```python
from build123d import *

# Parameters (mm, degrees)
MODEL_R                 = 1.25
BOSS_EXTRUDE1_DEPTH     = 2
BOSS_EXTRUDE2_DEPTH     = 11.50072
SKETCH2_R               = 1.25
CUT_EXTRUDE1_DEPTH      = 2
CUT_EXTRUDE1_DEPTH_BACK = 4


with BuildPart() as part:
    # Model → Boss-Extrude1 (new body)
    with BuildSketch(Plane.XY):
        Polygon((1.25, 4), (0, 4), (0, 8), (1.25, 8), (1.25, 12), (10.25072, 12), (10.25072, 8), (11.50072, 8), (11.50072, 4), (10.25072, 4), (10.25072, 0), (1.25, 0), align=None)
        with Locations((7.75072, 6)):
            Circle(MODEL_R, mode=Mode.SUBTRACT)
        with Locations((3.75, 6)):
            Circle(MODEL_R, mode=Mode.SUBTRACT)
    extrude(amount=BOSS_EXTRUDE1_DEPTH)

    # Sketch1 → Boss-Extrude2 (add)
    with BuildSketch(Plane.ZY):
        with BuildLine():
            Line((2, 4), (2, 5))
            ThreePointArc((2, 5), (2.292893219, 4.292893219), (3, 4))
            Line((3, 4), (2, 4))
        make_face()
        with BuildLine():
            Line((0, 4), (-1, 4))
            ThreePointArc((-1, 4), (-0.292893219, 4.292893219), (0, 5))
            Line((0, 5), (0, 4))
        make_face()
    extrude(amount=-BOSS_EXTRUDE2_DEPTH)

    # Sketch2 → Cut-Extrude1 (cut, two sides)
    with BuildSketch(Plane.XY.offset(2)) as cut_extrude1_sk:
        with Locations((3.75, 6)):
            Circle(SKETCH2_R)
        with Locations((7.75072, 6)):
            Circle(SKETCH2_R)
    extrude(amount=CUT_EXTRUDE1_DEPTH, mode=Mode.SUBTRACT)
    extrude(cut_extrude1_sk.sketch, amount=-CUT_EXTRUDE1_DEPTH_BACK, mode=Mode.SUBTRACT)


solid = part.part
```
Geometry: final body of the model. Coordinates: model frame, mm. A direction names the side the tool comes from. Round coordinates to 2 decimals unless told otherwise and drop trailing zeros. Write each loop counter-clockwise with the first axis right and the second up, starting at its lowest first coordinate (ties: lowest second). Pieces come first, ordered by that corner, then holes. Notation, with made-up numbers: (35, 71) -> (64, 71) arc R15 cw to (64, 75) -> close; hole circle Ø2 at (47.5, 38). An arc over 180 degrees is marked (long way). Return JSON: item names as keys, results as strings.
Q1. Set-up query: faces 1 (the flat face through (1.25, 10, 1)), 2 (the flat face through (6, 2, 2)), 3 (the flat face through (10.251, 2, 1)), 4 (the flat face through (6, 9, 2)), 5 (the flat face through (11, 8, 1)). Return all of +Z, -Z, +X, -X, +Y, -Y with unobstructed straight access to the full face (end or side cutting, diameter ignored); none if empty.
From the geometry:
{"face 1": "+Z, -Z, -X, +Y", "face 2": "+Z, +X, -X, -Y", "face 3": "+Z, -Z, +X, -Y", "face 4": "+Z, +X, -X, +Y", "face 5": "+Z, -Z, +X, +Y"}
Q2. Section C-C on z = 0.7. Return the cut outline in (x, y), and give its area (3 significant figures).
From the geometry:
{"outline": "(0, 4) -> (1.25, 4) -> (1.25, 0) -> (10.25, 0) -> (10.25, 4) -> (11.5, 4) -> (11.5, 8) -> (10.25, 8) -> (10.25, 12) -> (1.25, 12) -> (1.25, 8) -> (0, 8) -> close; hole circle Ø2.5 at (3.75, 6); hole circle Ø2.5 at (7.75, 6)", "area": "108 mm2"}
Q3. Mould query, pull axis Y, two halves, no side actions, for faces 6 (the cylindrical face through (4.327, 4.891, 0.986)), 7 (the flat face through (0, 6, 1)), 8 (the cylindrical face through (7, 5, 1)), 9 (the flat face through (1, 8, 1)). Classes: +Y half, -Y half, draft (parallel to the pull), parting line (faces both ways), or undercut.
From the geometry:
{"face 6": "undercut", "face 7": "draft", "face 8": "undercut", "face 9": "+Y half"}
Q4. Ray query, line 1 (X direction, y = 6, z = 0.7); line 2 (Y direction, x = 3.75, z = 0.65); line 3 (Z direction, x = 3.5, y = 3.75). Return the intervals inside material, ascending.
From the geometry:
{"line 1": "0 to 2.5, 5 to 6.5, 9 to 11.5", "line 2": "0 to 4.75, 7.25 to 12", "line 3": "0 to 2"}
Q5. Section A-A on y = 6. Return the cut outline in (x, z).
From the geometry:
{"outline": "(0, 0) -> (2.5, 0) -> (2.5, 2) -> (0, 2) -> close; (5, 0) -> (6.5, 0) -> (6.5, 2) -> (5, 2) -> close; (9, 0) -> (11.5, 0) -> (11.5, 2) -> (9, 2) -> close"}
Q6. Section D-D on x = 1.75. Return the cut outline in (y, z), and give its area (3 significant figures).
From the geometry:
{"outline": "(0, 0) -> (4, 0) -> (4, -1) arc R1 cw to (5, 0) -> (12, 0) -> (12, 2) -> (5, 2) arc R1 cw to (4, 3) -> (4, 2) -> (0, 2) -> close", "area": "24.4 mm2"}
Q7. Section B-B on x = 3.75. Return the cut outline in (y, z), and give its area (3 significant figures).
From the geometry:
{"outline": "(0, 0) -> (4, 0) -> (4, -1) arc R1 cw to (4.75, -0.03) -> (4.75, 2.03) arc R1 cw to (4, 3) -> (4, 2) -> (0, 2) -> close; (7.25, 0) -> (12, 0) -> (12, 2) -> (7.25, 2) -> close", "area": "19.4 mm2"}
Q8. First-contact query: pin 1 Ø1.6 at (y, z) = (11, 1) entering from +X; pin 2 Ø1.6 at (y, z) = (10, 1) entering from -X; pin 3 Ø2 at (x, z) = (4.5, 2.5) entering from -Y; pin 4 Ø5.5 at (x, y) = (7, 8.5) entering from -Z. Flat tips, straight axial feed; report the tip coordinate or a pass-through.
From the geometry:
{"pin 1": "x = 10.25", "pin 2": "x = 1.25", "pin 3": "y = 0", "pin 4": "z = 0"}
